from build123d import *

# Parameters (mm, degrees)
SKETCH1_R           = 1.7
BOSS_EXTRUDE1_DEPTH = 1.6


with BuildPart() as part:
    # Sketch1 → Boss-Extrude1 (new body)
    with BuildSketch(Plane(origin=(0, 0, 0), x_dir=(1, 0, 0), z_dir=(0, 1, 0))):
        Polygon((98.6, 0), (98.6, 2.6), (101.4, 5.4), (101.4, 37.6), (98.6, 40.4), (98.6, 51.9), (97.3, 53.2), (0, 53.2), (0, 0), align=None)
        with Locations(Location((95.9, 2.7, 0), (0, 0, 270))):
            Circle(SKETCH1_R, mode=Mode.SUBTRACT)
        with Locations(Location((89.8, 50.6, 0), (0, 0, 270))):
            Circle(SKETCH1_R, mode=Mode.SUBTRACT)
        with Locations(Location((65.95, 35.4, 0), (0, 0, 270))):
            Circle(SKETCH1_R, mode=Mode.SUBTRACT)
        with Locations(Location((65.95, 7.7, 0), (0, 0, 270))):
            Circle(SKETCH1_R, mode=Mode.SUBTRACT)
        with Locations(Location((15.35, 50.7, 0), (0, 0, 270))):
            Circle(SKETCH1_R, mode=Mode.SUBTRACT)
        with Locations(Location((14.1, 2.7, 0), (0, 0, 270))):
            Circle(SKETCH1_R, mode=Mode.SUBTRACT)
    extrude(amount=BOSS_EXTRUDE1_DEPTH)


solid = part.part
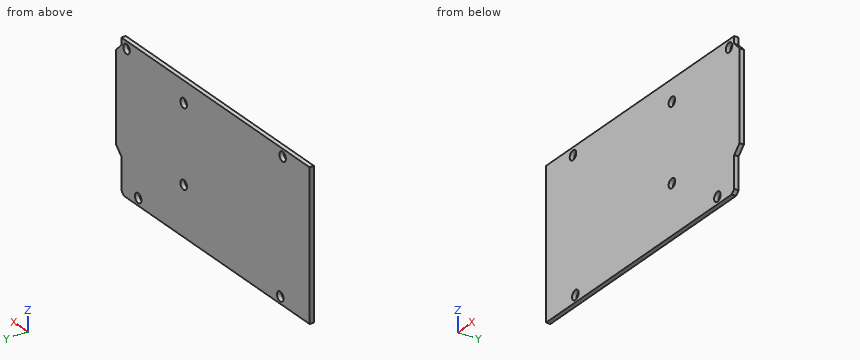
Work out the finished part from the listing and answer in its coordinate system (mm). Round coordinates to 2 decimals unless told otherwise and drop trailing zeros. Loops run counter-clockwise (first coordinate to the right, second up) from the corner with the lowest first, then second, coordinate; pieces in that order, holes last. Notation, with made-up numbers: (-23, 49) -> (-4, 49) arc R22 ccw to (-4, 71) -> close; hole circle Ø3 at (64.25, 77.25). An arc over 180 degrees is marked (long way). Use one line per item in the form item = value.
(1) Flat-ended cylindrical pins translate along their axes: P1, Ø4.5, axis at x = 14.1, z = -2.7, coming from the +Y side; P2, Ø0.5, axis at y = 1, z = -49, coming from the +X side. Find the tip coordinate at first contact, or state that the pin passes through.
Answer list:
P1 = 1.6
P2 = 98.6
(2) Find section A-A on x = 65.95. Give the vertices of the cut face in (y, z).
Answer list:
outline = (0, -53.2) -> (1.6, -53.2) -> (1.6, -37.1) -> (0, -37.1) -> close; (0, -33.7) -> (1.6, -33.7) -> (1.6, -9.4) -> (0, -9.4) -> close; (0, -6) -> (1.6, -6) -> (1.6, 0) -> (0, 0) -> close
(3) Find section D-D on y = 1. Give the vertices of the cut face in (x, z).
Answer list:
outline = (0, -53.2) -> (97.3, -53.2) -> (98.6, -51.9) -> (98.6, -40.4) -> (101.4, -37.6) -> (101.4, -5.4) -> (98.6, -2.6) -> (98.6, 0) -> (0, 0) -> close; hole circle Ø3.4 at (14.1, -2.7); hole circle Ø3.4 at (15.35, -50.7); hole circle Ø3.4 at (65.95, -35.4); hole circle Ø3.4 at (65.95, -7.7); hole circle Ø3.4 at (89.8, -50.6); hole circle Ø3.4 at (95.9, -2.7)
(4) Find section B-B on z = -7.7. Give the vertices of the cut face in (x, y), then the cut area to 3 significant figures.
Answer list:
outline = (0, 0) -> (64.25, 0) -> (64.25, 1.6) -> (0, 1.6) -> close; (67.65, 0) -> (101.4, 0) -> (101.4, 1.6) -> (67.65, 1.6) -> close
area = 157 mm2
(5) Find section C-C on x = 89.8. Give the vertices of the cut face in (y, z), then the cut area to 3 significant figures.
Answer list:
outline = (0, -53.2) -> (1.6, -53.2) -> (1.6, -52.3) -> (0, -52.3) -> close; (0, -48.9) -> (1.6, -48.9) -> (1.6, 0) -> (0, 0) -> close
area = 79.7 mm2
(6) Straight lines are drawn through the part: line 1 (Z direction, x = 65.95, y = 0.55); line 2 (Z direction, x = 95.9, y = 1.1); line 3 (Z direction, x = 89.8, y = 0.35). For each, find the intervals that lie inside material, in ascending order.
Answer list:
line_1 = -53.2 to -37.1, -33.7 to -9.4, -6 to 0
line_2 = -53.2 to -4.4, -1 to 0
line_3 = -53.2 to -52.3, -48.9 to 0
